Design review of the part built by this model. Coordinates are the model's own, in mm. Face numbers are marked on the shaded views. A direction names the side the tool comes from. Coordinates: 2 decimals unless noted, no trailing zeros. Loops run counter-clockwise (first coordinate to the right, second up) from the corner with the lowest first, then second, coordinate; pieces in that order, holes last. Notation, with made-up numbers: (46.25, 47) -> (97.25, 47) arc R27 ccw to (97.25, 76) -> close; hole circle Ø7 at (55.25, 56). An arc over 180 degrees is marked (long way). Use a Markdown table: item, result. Add a question column.
Q1. Clearance check with flat-ended pins moving along their axes: pin 1 Ø3.5 at (x, y) = (0, 0) entering from +Z; pin 2 Ø1 at (x, z) = (-10, 1) entering from +Y; pin 3 Ø1.5 at (x, z) = (-3, 3.5) entering from +Y. State where each tip first meets the part, or that it passes through.
Q2. Take a section at D-D on z = 2.3. Write out the cut boundary in (x, y).
Q3. For probe 1 along Y at (x, z) = (0, 2.15); probe 2 along Y at (x, z) = (0, 4.6), list the stretches that pass through material, from the lowest coordinate up.
Q4. Take a section at C-C on z = 3.85. Write out the cut boundary in (x, y), plus the area to 3 significant figures.
Q5. Draft analysis for pull direction Y (two halves, no side actions). For the marked faces 1, 2 and 3, state which applies: pulls with the +Y half, pulls with the -Y half, needs draft (parallel to the pull), parting line crosses it, or undercut.
Q6. For the marked faces 4 and 5, list the 3-axis set-ups (+Z, -Z, +X, -X, +Y, -Y) from which the entire face can be reached by the end or side of a thin tool; tool diameter is ignored.
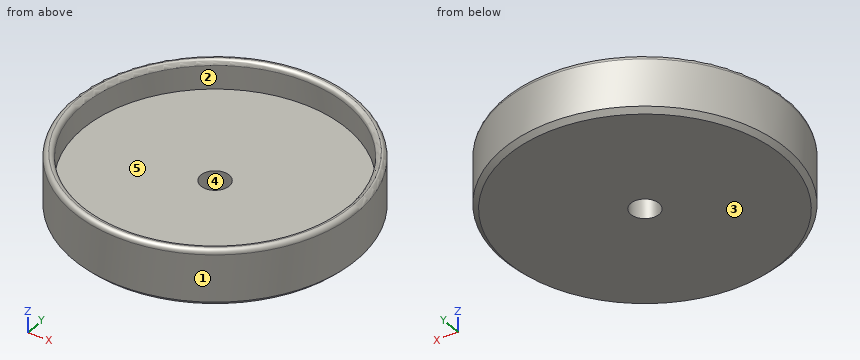
Autodesk Inventor part; units mm, degrees
ref_plane "YZ Plane" through (0, 0, 0) normal (1, 0, 0) x (0, 1, 0)
ref_plane "XZ Plane" through (0, 0, 0) normal (0, 1, 0) x (-1, 0, 0)
ref_plane "XY Plane" through (0, 0, 0) normal (0, 0, 1) x (1, 0, 0)
sketch "Sketch1" plane through (0, 0, 0) normal (1, 0, 0) x (0, 1, 0)
  line L0 (0, 0) -> (0, 6)
  line L1 (0, 6) -> (14, 6) construction
  line L2 (14, 6) -> (15, 6)
  line L3 (15, 6) -> (15, 0)
  line L4 (15, 0) -> (0, 0)
  line L5 (14, 6) -> (14, 3)
  line L6 (14, 3) -> (0, 3)
  dimension "d0" = 30
  dimension "d1" = 6
  dimension "d2" = 3
  dimension "d3" = 1
revolve "Revolution1" add sketch "Sketch1" angle 360 about axis through (0, 0, 0) along (0, 0, 1)
chamfer "Chamfer1" distance 0.5 angle 45 1 edges at (0, -15, 0)
sketch "Sketch2" plane through (0, 0, 0) normal (0, 0, -1) x (-1, 0, 0)
  point P0 (0, 0)
  point P1 (0, 0)
hole "Hole1" at (0, 0, 0) direction (0, 0, 1) diameter 3 end through all
thread "Thread1"
fillet "Fillet1" radius 0.5 2 edges at (0, -15, 6) (0, -14, 6)
properties part number "boron-bowl" material "Stainless Steel"
Answer list:
| question | item | result |
|---|---|---|
| 1 | pin 1 | z = 3 |
| 1 | pin 2 | y = 11.61 |
| 1 | pin 3 | y = 14.83 |
| 2 | outline | circle Ø30 at (0, 0); hole circle Ø3 at (0, 0) |
| 3 | probe 1 | -15 to -1.5, 1.5 to 15 |
| 3 | probe 2 | -15 to -14, 14 to 15 |
| 4 | outline | circle Ø30 at (0, 0); hole circle Ø28 at (0, 0) |
| 4 | area | 91.1 mm² |
| 5 | face 1 | parting line crosses it |
| 5 | face 2 | undercut |
| 5 | face 3 | needs draft |
| 6 | face 4 | +Z, -Z |
| 6 | face 5 | +Z |
